Autodesk Inventor part; units mm, degrees
ref_plane "YZ Plane" through (0, 0, 0) normal (1, 0, 0) x (0, 1, 0)
ref_plane "XZ Plane" through (0, 0, 0) normal (0, 1, 0) x (-1, 0, 0)
ref_plane "XY Plane" through (0, 0, 0) normal (0, 0, 1) x (1, 0, 0)
sketch "Sketch1" plane through (0, 0, 0) normal (0, 1, 0) x (-1, 0, 0)
  arc A0 (32.1154, 16) -> (30.1154, 14) centre (32.1154, 14) ccw
  line L0 (30.1154, 14) -> (30.1154, 10.91)
  line L1 (30.1154, 10.91) -> (-30.1154, 10.91)
  line L2 (-30.1154, 14) -> (-30.1154, 10.91)
  arc A1 (-30.1154, 14) -> (-32.1154, 16) centre (-32.1154, 14) ccw
  line L3 (-109, 16) -> (-32.1154, 16)
  arc A2 (-109, 16) -> (-111, 14) centre (-109, 14) ccw
  line L4 (-111, 14) -> (-111, -16.0875)
  arc A3 (-127.2776, -54.7893) -> (-111, -16.0875) centre (-158.9474, -18.6953) ccw
  line L5 (-127.2776, -54.7893) -> (-140.2776, -54.7893)
  arc A4 (-140.2776, -54.7893) -> (-152.2776, -66.7893) centre (-140.2776, -66.7893) ccw
  line L6 (-152.2776, -66.7893) -> (-152.2776, -304)
  arc A5 (-152.2776, -304) -> (-140.2776, -316) centre (-140.2776, -304) ccw
  line L7 (146.9429, -316) -> (-140.2776, -316)
  arc A6 (146.9429, -316) -> (158.9429, -304) centre (146.9429, -304) ccw
  line L8 (158.9429, -66.7893) -> (158.9429, -304)
  arc A7 (158.9429, -66.7893) -> (146.9429, -54.7893) centre (146.9429, -66.7893) ccw
  line L9 (126.134, -54.7893) -> (146.9429, -54.7893)
  arc A8 (111, -16.0875) -> (126.134, -54.7893) centre (168.0523, -16.0875) ccw
  line L10 (111, 14) -> (111, -16.0875)
  arc A9 (111, 14) -> (109, 16) centre (109, 14) ccw
  line L11 (109, 16) -> (32.1154, 16)
  circle A10 centre (44.6644, 1) radius 1.5
  circle A11 centre (70.3321, -126) radius 1.5
  circle A12 centre (70.3321, -296) radius 1.5
  circle A13 centre (-44.6644, 1) radius 1.5
  circle A14 centre (-70.3321, -296) radius 1.5
  circle A15 centre (-70.3321, -211) radius 1.5
  circle A16 centre (-70.3321, -126) radius 1.5
  circle A17 centre (-70.3321, -41) radius 1.5
  circle A18 centre (-138.2776, -61) radius 1.5
  circle A19 centre (-138.2776, -306) radius 1.5
  circle A20 centre (146.7224, -306) radius 1.5
  circle A21 centre (5.6569, -5.6569) radius 1.5
  circle A22 centre (-5.6569, -5.6569) radius 1.5
  circle A23 centre (-5.6569, 5.6569) radius 1.5
  circle A24 centre (5.6569, 5.6569) radius 1.5
  circle A25 centre (83.6863, -11.3137) radius 2
  circle A26 centre (0, 0) radius 5.25
  circle A27 centre (-95, 0) radius 6.75
  circle A28 centre (95, 0) radius 6.75
  circle A29 centre (146.7224, -61) radius 1.5
  circle A30 centre (-83.6863, 11.3137) radius 2
  circle A31 centre (-106.3137, 11.3137) radius 2
  circle A32 centre (-83.6863, -11.3137) radius 2
  circle A33 centre (-106.3137, -11.3137) radius 2
  circle A34 centre (106.3137, -11.3137) radius 2
  circle A35 centre (83.6863, 11.3137) radius 2
  circle A36 centre (70.3321, -211) radius 1.5
  circle A37 centre (70.3321, -41) radius 1.5
  circle A38 centre (106.3137, 11.3137) radius 2
  point P0 (0, 0)
extrude "Extrusion1" add sketch "Sketch1" along normal blind 6
properties part number "base da mesa de impressao"
The model under review builds one solid part; all positions refer to its coordinate system, in mm. Round coordinates to 2 decimals unless told otherwise and drop trailing zeros. Loops run counter-clockwise (first coordinate to the right, second up) from the corner with the lowest first, then second, coordinate; pieces in that order, holes last. Notation, with made-up numbers: (63.5, 48) - (74.5, 48) arc R22 ccw to (74.5, 80) - close; hole circle Ø9 at (65.5, -9). An arc over 180 degrees is marked (long way). Use CSV: the item, a comma, the result in double quotes.
(1) Take a section at C-C, the plane x = -23.5. Give the boundary of the cut face in (y, z), plus the area to 3 significant figures.
Working result:
outline,"(0, -316) - (6, -316) - (6, 10.91) - (0, 10.91) - close"
area,"1,960 mm^2"
(2) Clearance check with flat-ended pins moving along their axes: P1, Ø1.5, axis at y = 2.5, z = 13, coming from the -X side; P2, Ø1.8, axis at x = -141.5, y = 3.5, coming from the +Z side. State where each tip first meets the part, or that it passes through.
Working result:
P1,"stops at x = -111"
P2,"stops at z = -54.79"
(3) Take a section at B-B, the plane y = 1.2. State how many separate pieces and enclosed holes the cut face has, plus the area to 3 significant figures.
Working result:
separate pieces,"1"
enclosed holes,"29"
area,"96,300 mm^2"
(4) The part is to be moulded in two halves that separate along X. For faces 1 (the cylindrical face through (-5, 3, -1.6)), 2 (the cylindrical face through (-155.52, 2.96, -312.39)), 3 (the cylindrical face through (148.669, 2.958, -312.578)), say which applies: pulls with the +X half, pulls with the -X half, needs draft (parallel to the pull), parting line crosses it, or undercut.
Working result:
face 1,"undercut"
face 2,"pulls with the -X half"
face 3,"pulls with the +X half"
(5) For line 1 (X direction, y = 1.15, z = -2); line 2 (X direction, y = 0.4, z = -125.5); line 3 (Z direction, x = 82, y = 4.75), list the stretches that pass through material, from the lowest coordinate up.
Working result:
line 1,"x = -111 to -101.45, -88.55 to -4.85, 4.85 to 88.55, 101.45 to 111"
line 2,"x = -158.94 to -71.75, -68.92 to 68.92, 71.75 to 152.28"
line 3,"z = -316 to -12.39, -10.24 to 10.24, 12.39 to 16"
(6) Take a section at A-A, the plane x = -95. Give the boundary of the cut face in (y, z), plus the area to 3 significant figures.
Working result:
outline,"(0, -316) - (6, -316) - (6, -6.75) - (0, -6.75) - close; (0, 6.75) - (6, 6.75) - (6, 16) - (0, 16) - close"
area,"1,910 mm^2"
(7) Take a section at D-D, the plane x = 121. Give the boundary of the cut face in (y, z).
Working result:
outline,"(0, -316) - (6, -316) - (6, -48.12) - (0, -48.12) - close"
